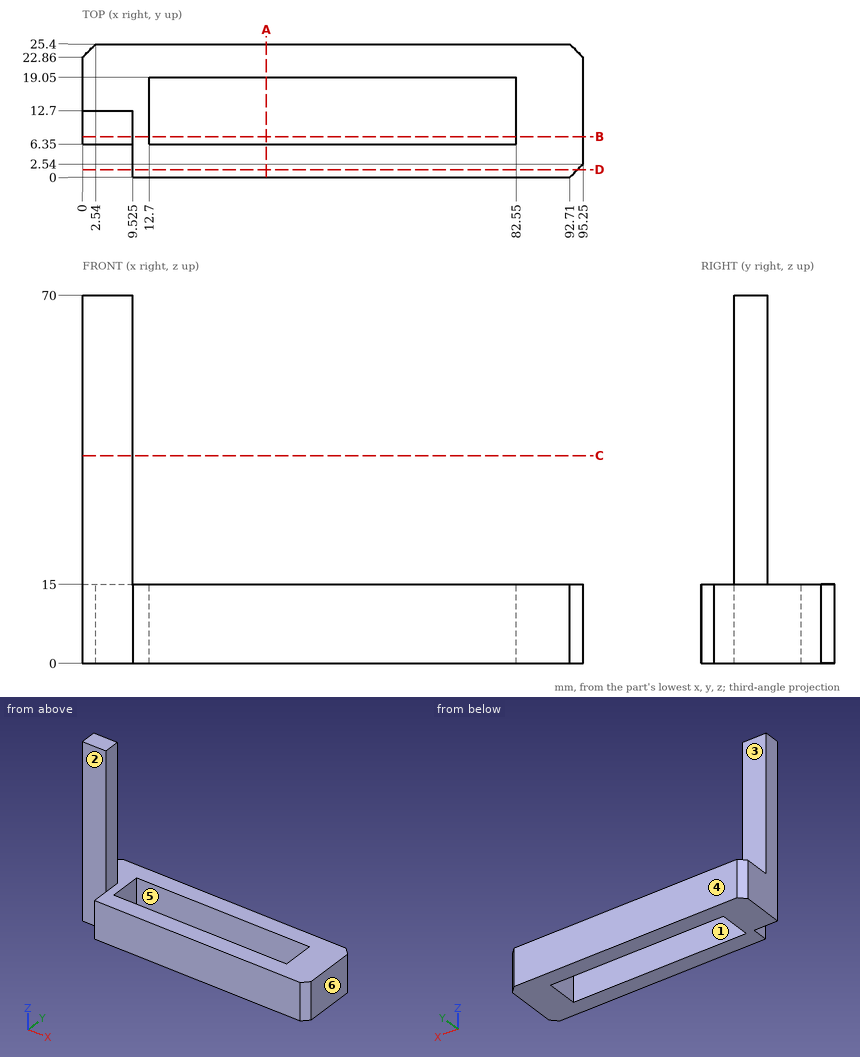
Answer from the drawing. Dimensions are ordinates in mm from the lowest x, y and z of the part. A direction names the side the tool comes from. Coordinates: 2 decimals unless noted, no trailing zeros. Loops run counter-clockwise (first coordinate to the right, second up) from the corner with the lowest first, then second, coordinate; pieces in that order, holes last. Notation, with made-up numbers: (28.5, -23.75) -> (87.5, -23.75) arc R15 ccw to (87.5, -4.75) -> close; hole circle Ø3 at (-38.5, 11.25). An arc over 180 degrees is marked (long way). Answer in a Markdown table with one row per item.
Item 1: For a pull along Y with two mould halves and no side action, classify the marked faces 4, 5 and 6 as released by +Y, released by -Y, zero draft, split by the parting line, or undercut.
Returned:
| item | result |
|---|---|
| face 4 | released by +Y |
| face 5 | undercut |
| face 6 | zero draft |
Item 2: A cutting plane is placed at D-D on y = 1.5. Determine the outline of the cut face in (x, z) (3 decimals), plus the area to 3 significant figures.
Returned:
| item | result |
|---|---|
| outline | (9.525, 0) -> (94.21, 0) -> (94.21, 15) -> (9.525, 15) -> close |
| area | 1,270 mm^2 |
Item 3: A cutting plane is placed at A-A on x = 35. Determine the outline of the cut face in (y, z).
Returned:
| item | result |
|---|---|
| outline | (0, 0) -> (6.35, 0) -> (6.35, 15) -> (0, 15) -> close; (19.05, 0) -> (25.4, 0) -> (25.4, 15) -> (19.05, 15) -> close |
Item 4: Straight lines are drawn through the part: line 1 along X through (y, z) = (6.75, 9); line 2 along Y through (x, z) = (49, 9.5); line 3 along X through (y, z) = (12.5, 63) (3 decimals). For each, find the intervals that lie inside material, in ascending order. Write a range as [from, to].
Returned:
| item | result |
|---|---|
| line 1 | x = [0, 12.7], [82.55, 95.25] |
| line 2 | y = [0, 6.35], [19.05, 25.4] |
| line 3 | x = [0, 9.525] |
Item 5: A cutting plane is placed at C-C on z = 39.5. Determine the outline of the cut face in (x, y) (3 decimals).
Returned:
| item | result |
|---|---|
| outline | (0, 6.35) -> (9.525, 6.35) -> (9.525, 12.7) -> (0, 12.7) -> close |
Item 6: A cutting plane is placed at B-B on y = 7.75. Determine the outline of the cut face in (x, z) (3 decimals).
Returned:
| item | result |
|---|---|
| outline | (0, 0) -> (12.7, 0) -> (12.7, 15) -> (9.525, 15) -> (9.525, 70) -> (0, 70) -> close; (82.55, 0) -> (95.25, 0) -> (95.25, 15) -> (82.55, 15) -> close |
Item 7: For the marked faces 1, 2 and 3, determine the directions among +Z, -Z, +X, -X, +Y, -Y from which every point of the face is accessible in a straight line to the end or side of a thin tool.
Returned:
| item | result |
|---|---|
| face 1 | +Z, -Z |
| face 2 | +Z, -Z, -X, -Y |
| face 3 | +Z, +X, -X, +Y |
Item 8: Each of these flat-tipped pins is pushed along its axis until it touches: P1, Ø8, axis at x = 65.5, y = 17.5, coming from the +Z side; P2, Ø1.9, axis at y = 10.5, z = 40, coming from the +X side (3 decimals); P3, Ø7.5, axis at x = 5.5, z = 22.5, coming from the -Y side; P4, Ø2, axis at x = 78, y = 22, coming from the -Z side. Where does it stop, or does it pass through?
Returned:
| item | result |
|---|---|
| P1 | stops at z = 15 |
| P2 | stops at x = 9.525 |
| P3 | stops at y = 6.35 |
| P4 | stops at z = 0 |
